from build123d import *

# Parameters (mm, degrees)
F0_W     = 9.906
F0_H     = 36.322
F1_DEPTH = 5.08
F2_R     = 1.124354
F3_DEPTH = 25.4


with BuildPart() as f1:
    # F0 (on Front) → F1 (new body)
    with BuildSketch(Plane.XZ):
        Polygon((-7.89122, 0), (-4.869051, 0), (0, 0), (7.89122, 0), (7.89122, 40.64), (-7.89122, 40.64), align=None)
        with Locations((0.083949, 20.794085)):
            Rectangle(F0_W, F0_H, mode=Mode.SUBTRACT)
    extrude(amount=F1_DEPTH)

    # F2 (on face) → F3 (cut)
    with BuildSketch(Plane.YZ.offset(7.89122)):
        with Locations((-2.54, 40.64)):
            Circle(F2_R)
    extrude(amount=-F3_DEPTH, mode=Mode.SUBTRACT)


solid = f1.part
For this review, take the finished solid that the model builds, in its own axes (mm). A direction names the side the tool comes from. Round coordinates to 2 decimals unless told otherwise and drop trailing zeros. Write each loop counter-clockwise with the first axis right and the second up, starting at its lowest first coordinate (ties: lowest second). Pieces come first, ordered by that corner, then holes. Notation, with made-up numbers: (33.25, 47) - (50.25, 47) arc R13 ccw to (50.25, 67) - close; hole circle Ø11 at (20, -37.75). An arc over 180 degrees is marked (long way). Write item = value, one per line. Start each with the question number.
1. Consider section C-C on x = 1.5. State the section outline as (y, z) points, plus the area to 3 significant figures.
2. Wall thickness on L1, parallel to X at y = -2.3, z = 34; L2, parallel to Z at x = 3, y = -0.5; L3, parallel to Z at x = -0.5, y = -2.8: over which ranges is each line inside the solid? List them lowest first.
3. Draft analysis for pull direction Y (two halves, no side actions). For faces 3 (the face through (-4.869, -3, 21)), 4 (the face through (0.11, -2.565, 39.516)), 5 (the face through (5.2, 0, 20.6)), state which applies: released by +Y, released by -Y, zero draft, split by the parting line, or undercut.
4. For pin 1 Ø8 at (x, z) = (0, 33) entering from -Y; pin 2 Ø2.5 at (x, y) = (-1.5, -2) entering from +Z, all flat-tipped, find the tip position at first contact; note any pin that passes through.
5. For faces 1 (the face through (0, -3, 2.633)), 2 (the face through (0, -3, 0)), list the 3-axis set-ups (+Z, -Z, +X, -X, +Y, -Y) from which the entire face can be reached by the end or side of a thin tool; tool diameter is ignored.
6. Consider section A-A on z = 18.5. State the section outline as (x, y) points.
7. Consider section B-B on y = -2.54. State the section outline as (x, z) points.
Evaluation:
q1.outline = (-5.08, 0) - (0, 0) - (0, 2.63) - (-5.08, 2.63) - close; (-5.08, 38.96) - (0, 38.96) - (0, 40.64) - (-1.42, 40.64) arc R1.12 cw to (-3.66, 40.64) - (-5.08, 40.64) - close
q1.area = 19.9 mm2
q2.L1 = -7.89 to -4.87, 5.04 to 7.89
q2.L2 = 0 to 2.63, 38.96 to 40.64
q2.L3 = 0 to 2.63, 38.96 to 39.55
q3.face_3 = zero draft
q3.face_4 = undercut
q3.face_5 = released by +Y
q4.pin_1 = through
q4.pin_2 = 40.64
q5.face_1 = +Y, -Y
q5.face_2 = -Z, +X, -X, +Y, -Y
q6.outline = (-7.89, -5.08) - (-4.87, -5.08) - (-4.87, 0) - (-7.89, 0) - close; (5.04, -5.08) - (7.89, -5.08) - (7.89, 0) - (5.04, 0) - close
q7.outline = (-7.89, 0) - (7.89, 0) - (7.89, 39.52) - (-7.89, 39.52) - close; hole (-4.87, 2.63) - (5.04, 2.63) - (5.04, 38.96) - (-4.87, 38.96) - close
